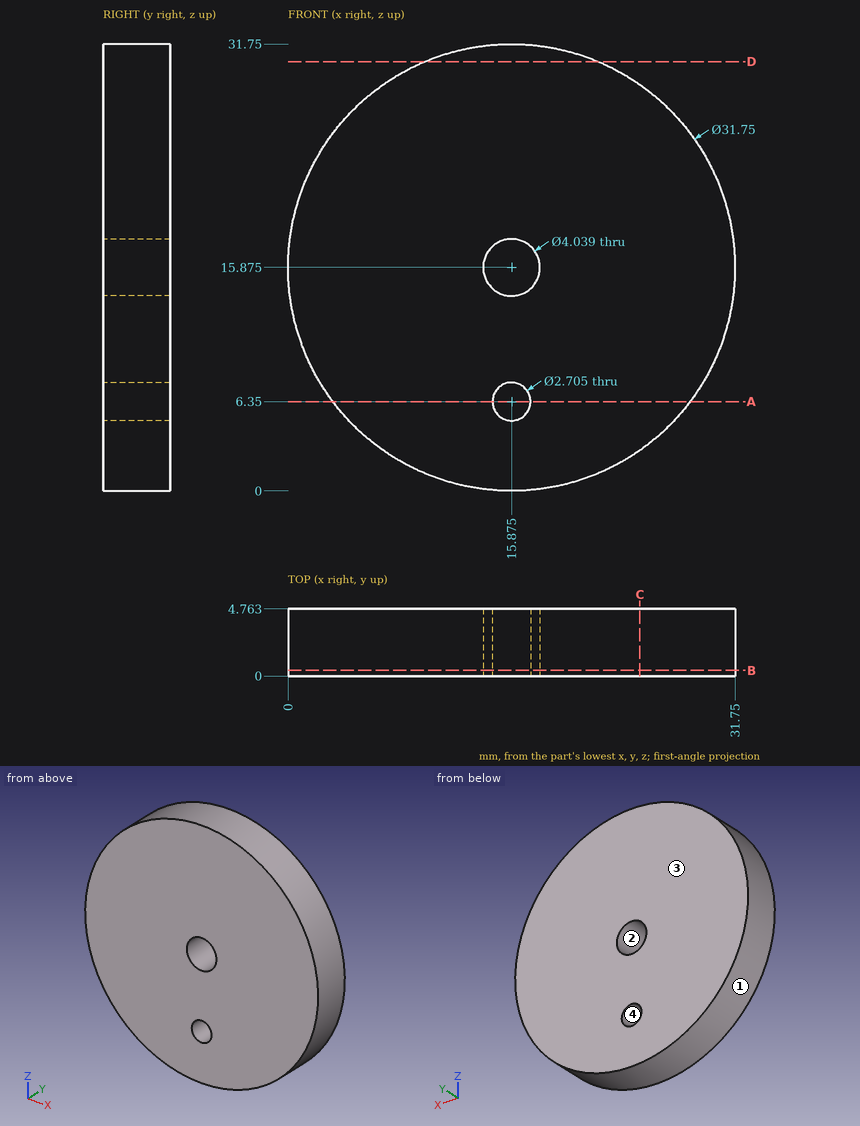
Input: dimensioned drawing with shaded views. Units: mm. Origin: part minimum x, y, z. Coordinates: 2 decimals unless noted, no trailing zeros. Loops run counter-clockwise (first coordinate to the right, second up) from the corner with the lowest first, then second, coordinate; pieces in that order, holes last. Notation, with made-up numbers: (-10, 7) -> (8, 7) arc R23 cw to (8, 46) -> close; hole circle Ø10 at (48, 82). An arc over 180 degrees is marked (long way). One line per item, written item: value. Start each with the question number.
Q1. Contact query for flat-ended pins moving along their axis: P1, Ø2, axis at y = 1.5, z = 11.5, coming from the +X side; P2, Ø1.5, axis at x = 13.5, y = 1, coming from the +Z side; P3, Ø1.5, axis at x = 19.5, y = 3.5, coming from the +Z side. Output: stop coordinate, or through.
Q2. Mould query, pull axis X, two halves, no side actions, for the marked faces 1, 2, 3 and 4. Classes: pulls with the +X half, pulls with the -X half, needs draft (parallel to the pull), parting line crosses it, or undercut.
Q3. Section query A-A, the plane z = 6.35. Return the cut outline in (x, y) (1 decimal), and give its area (3 significant figures).
Q4. Section query D-D, the plane z = 30.5. Return the cut outline in (x, y).
Q5. Line query: line 1 along X through (y, z) = (1.9, 17); line 2 along X through (y, z) = (2.5, 15) (1 decimal); line 3 along Z through (x, y) = (12.5, 1.95). Output: solid intervals per line, ascending.
Q6. Section query C-C, the plane x = 25. Return the cut outline in (y, z) (1 decimal).
Q7. Section query B-B, the plane y = 0.4. Give the number of separate pieces and of enclosed holes in the cut face, and give its area (3 significant figures).
Results:
1. P1: x = 31.39
1. P2: z = 31.67
1. P3: z = 31.49
2. face 1: parting line crosses it
2. face 2: undercut
2. face 3: needs draft
2. face 4: undercut
3. outline: (3.2, 0) -> (14.5, 0) -> (14.5, 4.8) -> (3.2, 4.8) -> close; (17.2, 0) -> (28.6, 0) -> (28.6, 4.8) -> (17.2, 4.8) -> close
3. area: 108 mm^2
4. outline: (9.7, 0) -> (22.05, 0) -> (22.05, 4.76) -> (9.7, 4.76) -> close
5. line 1: 0.04 to 14.2, 17.55 to 31.71
5. line 2: 0 to 14.1, 17.7 to 31.7
5. line 3: 0.36 to 31.39
6. outline: (0, 2.9) -> (4.8, 2.9) -> (4.8, 28.9) -> (0, 28.9) -> close
7. separate pieces: 1
7. enclosed holes: 2
7. area: 773 mm^2
